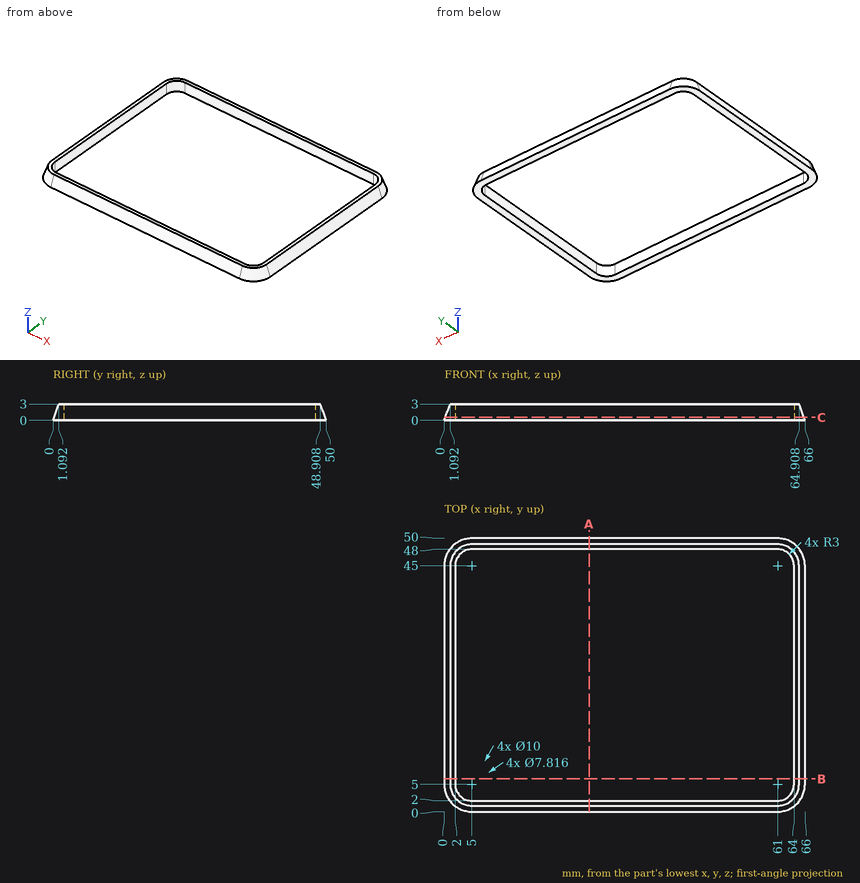
Input: dimensioned drawing with shaded views. Units: mm. Origin: part minimum x, y, z. Give positions to 0.01 mm unless a question says otherwise; leave off trailing zeros. Write each loop counter-clockwise with the first axis right and the second up, starting at its lowest first coordinate (ties: lowest second). Pieces come first, ordered by that corner, then holes.
1. Section query B-B (y = 6). Return the cut outline in (x, z).
2. Section query C-C (z = 0.55). Return the cut outline in (x, y), then the cut area to 3 significant figures.
3. Section query A-A (x = 26.5). Return the cut outline in (y, z).
4. First-contact query: pin 1 (1.5 mm diameter, centred on x = 28, z = 1, fed in from +Y); pin 2 (1.5 mm diameter, centred on x = 53.5, z = 2.5, fed in from +Y); pin 3 (12 mm diameter, centred on x = 30, y = 11, fed in from -Z); pin 4 (0.9 mm diameter, centred on y = 30.5, z = 1.5, fed in from -X). Flat tips, straight axial feed; report the tip coordinate or a pass-through.
5. Material intervals for line 1 along X through (y, z) = (6.5, 2.5); line 2 along Y through (x, z) = (4, 1.2); line 3 along Y through (x, z) = (49, 1.1), sorted ascending.
Output values:
1. outline: (0, 0) - (2, 0) - (2, 3) - (1.09, 3) - close; (64, 0) - (66, 0) - (64.91, 3) - (64, 3) - close
2. outline: (0.2, 5) arc R4.8 ccw to (5, 0.2) - (61, 0.2) arc R4.8 ccw to (65.8, 5) - (65.8, 45) arc R4.8 ccw to (61, 49.8) - (5, 49.8) arc R4.8 ccw to (0.2, 45) - close; hole (2, 5) arc R3 ccw to (5, 2) - (61, 2) arc R3 ccw to (64, 5) - (64, 45) arc R3 ccw to (61, 48) - (5, 48) arc R3 ccw to (2, 45) - close
2. area: 390 mm2
3. outline: (0, 0) - (2, 0) - (2, 3) - (1.09, 3) - close; (48, 0) - (50, 0) - (48.91, 3) - (48, 3) - close
4. pin 1: stops at y = 49.91
4. pin 2: stops at y = 49.36
4. pin 3: passes through
4. pin 4: stops at x = 0.38
5. line 1: x = 0.91 to 2, 64 to 65.09
5. line 2: y = 0.55 to 2.17, 47.83 to 49.45
5. line 3: y = 0.4 to 2, 48 to 49.6
